from build123d import *

# Parameters (mm, degrees)
EXTRUDE_1_DEPTH     = 432
CUT_EXTRUDE_5_DEPTH = 14
CUT_EXTRUDE_6_DEPTH = 14
CUT_EXTRUDE_7_DEPTH = 433.455778086
SKETCH_10_R         = 2.3
CUT_EXTRUDE_8_DEPTH = 433.455778086
CHAMFER_1_SIZE      = 2.05


with BuildPart() as part:
    # Эскиз1 → Бобышка-Вытянуть1 (new body)
    with BuildSketch(Plane(origin=(0, 0, 0), x_dir=(0, 0, -1), z_dir=(1, 0, 0))):
        with BuildLine():
            Line((0, 0), (0, 15))
            Line((0, 15), (1, 15))
            ThreePointArc((1, 15), (1.707106781, 14.707106781), (2, 14))
            Line((2, 14), (2, 3))
            ThreePointArc((2, 3), (2.292893219, 2.292893219), (3, 2))
            Line((3, 2), (14, 2))
            ThreePointArc((14, 2), (14.707106781, 1.707106781), (15, 1))
            Line((15, 1), (15, 0))
            Line((15, 0), (0, 0))
        make_face()
    extrude(amount=EXTRUDE_1_DEPTH)

    # Эскиз6 → Вырез-Вытянуть5 (cut)
    with BuildSketch(Plane(origin=(432, 0, 0), x_dir=(0, 0, -1), z_dir=(1, 0, 0))):
        Polygon((0, 15), (2, 15), (3, 15), (3, 2), (2, 2), (2, 0), (0, 0), align=None)
    extrude(amount=-CUT_EXTRUDE_5_DEPTH, mode=Mode.SUBTRACT)

    # Эскиз7 → Вырез-Вытянуть6 (cut)
    with BuildSketch(Plane.ZY):
        Polygon((0, 15), (-2, 15), (-3, 15), (-3, 2), (-2, 2), (-2, 0), (0, 0), align=None)
    extrude(amount=-CUT_EXTRUDE_6_DEPTH, mode=Mode.SUBTRACT)

    # Эскиз9 → Вырез-Вытянуть7 (cut, through all)
    with BuildSketch(Plane(origin=(0, 2, 0), x_dir=(1, 0, 0), z_dir=(0, 1, 0))):
        Polygon((0, 2), (0, 7), (5, 2), align=None)
        Polygon((432, 2), (432, 7), (427, 2), align=None)
    extrude(amount=-CUT_EXTRUDE_7_DEPTH, mode=Mode.SUBTRACT)

    # Эскиз10 → Вырез-Вытянуть8 (cut, through all)
    with BuildSketch(Plane(origin=(0, 2, 0), x_dir=(1, 0, 0), z_dir=(0, 1, 0))):
        with Locations(Location((40, 8, 0), (0, 0, 270))):
            Circle(SKETCH_10_R)
        with Locations(Location((392, 8, 0), (0, 0, 270))):
            Circle(SKETCH_10_R)
    extrude(amount=-CUT_EXTRUDE_8_DEPTH, mode=Mode.SUBTRACT)

    # Фаска1
    # the kernel refuses this chamfer: 2.05 mm, written as the material it takes off along each edge
    with BuildSketch(Plane(origin=(40, 2, -8), x_dir=(0, 0, 1), z_dir=(-1, 0, 0))) as chamfer_1_piece_1:
        Polygon((2.3 + CHAMFER_1_SIZE, 0), (2.3, -CHAMFER_1_SIZE), (2.3, 0), align=None)
    revolve(axis=Axis((40, 2, -8), (0, 1, 0)), mode=Mode.SUBTRACT)
    with BuildSketch(Plane(origin=(392, 2, -8), x_dir=(0, 0, 1), z_dir=(-1, 0, 0))) as chamfer_1_piece_2:
        Polygon((2.3 + CHAMFER_1_SIZE, 0), (2.3, -CHAMFER_1_SIZE), (2.3, 0), align=None)
    revolve(axis=Axis((392, 2, -8), (0, 1, 0)), mode=Mode.SUBTRACT)


solid = part.part
Could you check a few things on this model? Use its own coordinates, in mm. A direction names the side the tool comes from. Give positions to 0.01 mm unless a question says otherwise; leave off trailing zeros. Order: outer loops, then holes, each group sorted by start corner. A loop starts at its lowest first (then second) coordinate and runs counter-clockwise, first axis right, second up. Notation, with made-up numbers: (36, 38.25) - (68, 38.25) arc R10 cw to (68, 45.25) - close; hole circle Ø4 at (47, 87.25). An arc over 180 degrees is marked (long way). Return JSON: item names as keys, results as strings. Group by question number.
Q1. Which directions (+Z, -Z, +X, -X, +Y, -Y) give clear straight access to the entire face, cutting with the end or side of a thin tool? Please do faces 1 (the face through (213, 9, -2)), 2 (the face through (213, 0, -8)).
Q2. Suppose I cut it at A-A, the plane x = 392. Please give me the cut outline in (y, z), and give its area (3 significant figures).
Q3. Please list where these lines run through material, in increasing order: line 1 along X through (y, z) = (8.25, -1.75); line 2 along Y through (x, z) = (140, -10.5); line 3 along Z through (x, y) = (135, 4.5). Write a range as [from, to].
Q4. Will these pins go through, and if not, where does the flat tip stop? pin 1 Ø3 at (x, z) = (248.5, -10.5) entering from +Y; pin 2 Ø4 at (x, z) = (140, -12) entering from -Y; pin 3 Ø2 at (x, y) = (421.5, 1) entering from +Z; pin 4 Ø0.9 at (y, z) = (10.5, -1) entering from +X.
Q5. Suppose I cut it at B-B, the plane x = 250. Please give me the cut outline in (y, z), and give its area (3 significant figures).
Q6. Suppose I cut it at C-C, the plane y = 8.25. Please give me the cut outline in (x, z), and give its area (3 significant figures).
Resolved:
{
 "1": {"face 1": "-Z, +X, -X, +Y", "face 2": "+Z, -Z, +X, -X, -Y"},
 "2": {"outline": "(0, -15) - (1, -15) arc R1 ccw to (2, -14) - (2, -12.35) - (0, -10.35) - close; (0, -5.65) - (2, -3.65) - (2, -3) arc R1 cw to (3, -2) - (14, -2) arc R1 ccw to (15, -1) - (15, 0) - (0, 0) - close", "area": "42.4 mm2"},
 "3": {"line 1": "x = [14, 418]", "line 2": "y = [0, 2]", "line 3": "z = [-2, 0]"},
 "4": {"pin 1": "stops at y = 2", "pin 2": "stops at y = 0", "pin 3": "stops at z = -2", "pin 4": "stops at x = 418"},
 "5": {"outline": "(0, -15) - (1, -15) arc R1 ccw to (2, -14) - (2, -3) arc R1 cw to (3, -2) - (14, -2) arc R1 ccw to (15, -1) - (15, 0) - (0, 0) - close", "area": "55.8 mm2"},
 "6": {"outline": "(14, -2) - (418, -2) - (418, 0) - (14, 0) - close", "area": "808 mm2"}
}
